Work out the finished part from the listing and answer in its coordinate system (mm). Face numbers are marked on the shaded views. Coordinates: 2 decimals unless noted, no trailing zeros. Order: outer loops, then holes, each group sorted by start corner. A loop starts at its lowest first (then second) coordinate and runs counter-clockwise, first axis right, second up. Notation, with made-up numbers: M 45,33.25 L 78,33.25 A11 cw 78,41.25 Z; hole C -27,-39.5 d2. An arc over 180 degrees is marked long. Answer in a Markdown table with one row per item. Add a question column.
Item 1: The part is cut by section D-D (z = -15.5). Write down the section's boundary in (x, y), then the cut area to 3 significant figures.
Item 2: The part is cut by section A-A (x = 0). Write down the section's boundary in (y, z), then the cut area to 3 significant figures.
Item 3: Flat-ended cylindrical pins translate along their axes: pin 1 Ø4.5 at (x, z) = (0, 38) entering from +Y; pin 2 Ø4 at (x, y) = (27, -2) entering from +Z; pin 3 Ø4 at (x, y) = (3, 3) entering from +Z; pin 4 Ø1 at (y, z) = (-2.5, -16.5) entering from +X. Find the tip coordinate at first contact, or state that the pin passes through.
Item 4: The part is cut by section B-B (z = 38). Write down the section's boundary in (x, y), then the cut area to 3 significant figures.
Item 5: The part is cut by section C-C (x = -23). Write down the section's boundary in (y, z).
Item 6: The mould has two halves that part along X. Classify the marked faces 1 and 2: released by +X, released by -X, zero draft, split by the parting line, or undercut.
Item 7: Consider line 1 (Y direction, x = -30, z = 35.5); line 2 (X direction, y = -4.5, z = -28); line 3 (X direction, y = -1.5, z = 38). Determine where each line is inside the solid, lowest interval first. Write a range as from..to.
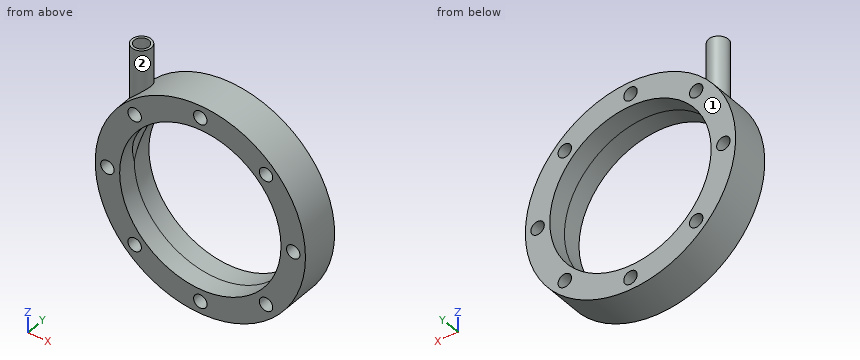
from build123d import *

# Parameters (mm, degrees)
SKETCH001_R           = 43
PAD_DEPTH             = 8
SKETCH002_W           = 4
SKETCH002_H           = 50
SKETCH003_R           = 33
POCKET_DEPTH          = 8.001
POCKET_DEPTH_BACK     = 8.001
SKETCH004_W           = 3
SKETCH004_H           = 50
SKETCH013_R           = 2.75
POCKET005_DEPTH       = 271.35174
POLARPATTERN003_COUNT = 8


with BuildPart() as part:
    # Sketch001 → Pad (new body, symmetric)
    with BuildSketch(Plane.XZ):
        Circle(SKETCH001_R)
    extrude(amount=PAD_DEPTH, both=True)

    # Sketch002 → Revolution (revolve)
    with BuildSketch(Plane.XZ):
        with Locations((-28, 25)):
            Rectangle(SKETCH002_W, SKETCH002_H)
    revolve(axis=Axis((-30, 0, 40.402922), (0, 0, 1)))

    # Sketch003 → Pocket (cut, two sides)
    with BuildSketch(Plane.XZ) as pocket_sk:
        Circle(SKETCH003_R)
    extrude(amount=-POCKET_DEPTH, mode=Mode.SUBTRACT)
    extrude(pocket_sk.sketch, amount=POCKET_DEPTH_BACK, mode=Mode.SUBTRACT)

    # Sketch004 → Groove (revolve, cut)
    with BuildSketch(Plane.XZ):
        with Locations((-31.5, 25)):
            Rectangle(SKETCH004_W, SKETCH004_H)
    revolve(axis=Axis((-30, 0, 22.276785), (0, 0, 1)), mode=Mode.SUBTRACT)

    # Sketch013 (on Face4 of Groove) → Pocket005 (cut, through all)
    with BuildSketch(Plane.XZ.offset(8)):
        with Locations((0, -38)):
            Circle(SKETCH013_R)
    pocket005 = extrude(amount=-POCKET005_DEPTH, mode=Mode.SUBTRACT)

    # PolarPattern003: Pocket005 ×8 about axis
    polarpattern003_axis = Axis((0, -8, 0), (0, -1, 0))
    for i in range(1, POLARPATTERN003_COUNT):
        add(pocket005.rotate(polarpattern003_axis, i * 360 / POLARPATTERN003_COUNT), mode=Mode.SUBTRACT)


solid = part.part
Reply:
| question | item | result |
|---|---|---|
| 1 | outline | M -40.11,-8 L -29.13,-8 L -29.13,8 L -40.11,8 Z; M 29.13,-8 L 40.11,-8 L 40.11,8 L 29.13,8 Z |
| 1 | area | 351 mm2 |
| 2 | outline | M -8,-43 L 8,-43 L 8,-40.75 L -8,-40.75 Z; M -8,-35.25 L 8,-35.25 L 8,-33 L -8,-33 Z; M -8,33 L 8,33 L 8,35.25 L -8,35.25 Z; M -8,40.75 L 8,40.75 L 8,43 L -8,43 Z |
| 2 | area | 144 mm2 |
| 3 | pin 1 | passes through |
| 3 | pin 2 | stops at z = 34.99 |
| 3 | pin 3 | stops at z = 42.99 |
| 3 | pin 4 | stops at x = 39.91 |
| 4 | outline | C -30,0 d8; M -20.12,-8 L -2.75,-8 L -2.75,8 L -20.12,8 Z; M 2.75,-8 L 20.12,-8 L 20.12,8 L 2.75,8 Z; hole C -30,0 d6 |
| 4 | area | 578 mm2 |
| 5 | outline | M -8,-36.33 L 8,-36.33 L 8,-23.66 L -8,-23.66 Z; M -8,23.66 L 8,23.66 L 8,36.33 L -8,36.33 Z |
| 6 | face 1 | zero draft |
| 6 | face 2 | undercut |
| 7 | line 1 | y = -4..-3, 3..4 |
| 7 | line 2 | x = -32.63..-29.38, -24.36..-17.46, 17.46..24.36, 29.38..32.63 |
| 7 | line 3 | x = -33.71..-32.6, -27.4..-26.29, -20.12..-2.75, 2.75..20.12 |
